Design review of the part built by this model. Coordinates are the model's own, in mm. Round coordinates to 2 decimals unless told otherwise and drop trailing zeros. Write each loop counter-clockwise with the first axis right and the second up, starting at its lowest first coordinate (ties: lowest second). Pieces come first, ordered by that corner, then holes. Notation, with made-up numbers: (20, 16) - (72, 16) arc R27 cw to (72, 53) - close; hole circle Ø9 at (57.25, 77). An arc over 180 degrees is marked (long way). Use one line per item in the form item = value.
```python
from build123d import *

# Parameters (mm, degrees)
SKETCH1_R           = 4.1656
BOSS_EXTRUDE1_DEPTH = 3.175
CUT_EXTRUDE2_DEPTH  = 104.862786526
FILLET1_R           = 12.7


with BuildPart() as part:
    # Sketch1 → Boss-Extrude1 (new body)
    with BuildSketch(Plane.XY):
        with BuildLine():
            Line((-93.98, 26.67), (93.98, 26.67))
            ThreePointArc((93.98, 26.67), (98.470128061, 24.810128061), (100.33, 20.32))
            Line((100.33, 20.32), (100.33, -20.32))
            ThreePointArc((100.33, -20.32), (98.470128061, -24.810128061), (93.98, -26.67))
            Line((93.98, -26.67), (-93.98, -26.67))
            ThreePointArc((-93.98, -26.67), (-98.470128061, -24.810128061), (-100.33, -20.32))
            Line((-100.33, -20.32), (-100.33, 20.32))
            ThreePointArc((-100.33, 20.32), (-98.470128061, 24.810128061), (-93.98, 26.67))
        make_face()
        with Locations((-78.74, 10.922)):
            Circle(SKETCH1_R, mode=Mode.SUBTRACT)
        with Locations((-78.74, -10.922)):
            Circle(SKETCH1_R, mode=Mode.SUBTRACT)
        with Locations(Location((78.74, -10.922, 0), (0, 0, 180))):
            Circle(SKETCH1_R, mode=Mode.SUBTRACT)
        with Locations(Location((78.74, 10.922, 0), (0, 0, 180))):
            Circle(SKETCH1_R, mode=Mode.SUBTRACT)
        with BuildLine():
            Line((-11.43, 13.97), (11.43, 13.97))
            ThreePointArc((11.43, 13.97), (13.226051224, 13.226051224), (13.97, 11.43))
            Line((13.97, 11.43), (13.97, -11.43))
            ThreePointArc((13.97, -11.43), (13.226051224, -13.226051224), (11.43, -13.97))
            Line((11.43, -13.97), (-11.43, -13.97))
            ThreePointArc((-11.43, -13.97), (-13.226051224, -13.226051224), (-13.97, -11.43))
            Line((-13.97, -11.43), (-13.97, 11.43))
            ThreePointArc((-13.97, 11.43), (-13.226051224, 13.226051224), (-11.43, 13.97))
        make_face(mode=Mode.SUBTRACT)
        with BuildLine():
            Line((-52.07, 3.556), (-49.53, 3.556))
            ThreePointArc((-49.53, 3.556), (-45.974, 0), (-49.53, -3.556))
            Line((-49.53, -3.556), (-52.07, -3.556))
            ThreePointArc((-52.07, -3.556), (-55.626, 0), (-52.07, 3.556))
        make_face(mode=Mode.SUBTRACT)
        with BuildLine():
            Line((-26.67, 3.556), (-24.13, 3.556))
            ThreePointArc((-24.13, 3.556), (-20.574, 0), (-24.13, -3.556))
            Line((-24.13, -3.556), (-26.67, -3.556))
            ThreePointArc((-26.67, -3.556), (-30.226, 0), (-26.67, 3.556))
        make_face(mode=Mode.SUBTRACT)
        with BuildLine():
            Line((26.67, 3.556), (24.13, 3.556))
            ThreePointArc((24.13, 3.556), (20.574, 0), (24.13, -3.556))
            Line((24.13, -3.556), (26.67, -3.556))
            ThreePointArc((26.67, -3.556), (30.226, 0), (26.67, 3.556))
        make_face(mode=Mode.SUBTRACT)
        with BuildLine():
            Line((52.07, 3.556), (49.53, 3.556))
            ThreePointArc((49.53, 3.556), (45.974, 0), (49.53, -3.556))
            Line((49.53, -3.556), (52.07, -3.556))
            ThreePointArc((52.07, -3.556), (55.626, 0), (52.07, 3.556))
        make_face(mode=Mode.SUBTRACT)
    extrude(amount=BOSS_EXTRUDE1_DEPTH)

    # Sketch3 → Cut-Extrude2 (cut, through all)
    with BuildSketch(Plane.XY):
        with BuildLine():
            Line((-71.12, 26.67), (-63.409743879, 18.959743879))
            ThreePointArc((-63.409743879, 18.959743879), (-59.289567349, 16.206729937), (-54.429487758, 15.24))
            Line((-54.429487758, 15.24), (-35.650256121, 15.24))
            ThreePointArc((-35.650256121, 15.24), (-30.79017653, 16.206729937), (-26.67, 18.959743879))
            Line((-26.67, 18.959743879), (-18.959743879, 26.67))
            Line((-18.959743879, 26.67), (-71.12, 26.67))
        make_face()
        with BuildLine():
            Line((-71.12, -26.67), (-18.959743879, -26.67))
            Line((-18.959743879, -26.67), (-26.67, -18.959743879))
            ThreePointArc((-26.67, -18.959743879), (-30.79017653, -16.206729937), (-35.650256121, -15.24))
            Line((-35.650256121, -15.24), (-54.429487758, -15.24))
            ThreePointArc((-54.429487758, -15.24), (-59.289567349, -16.206729937), (-63.409743879, -18.959743879))
            Line((-63.409743879, -18.959743879), (-71.12, -26.67))
        make_face()
        with BuildLine():
            Line((71.12, -26.67), (63.409743879, -18.959743879))
            ThreePointArc((63.409743879, -18.959743879), (59.289567349, -16.206729937), (54.429487758, -15.24))
            Line((54.429487758, -15.24), (35.650256121, -15.24))
            ThreePointArc((35.650256121, -15.24), (30.79017653, -16.206729937), (26.67, -18.959743879))
            Line((26.67, -18.959743879), (18.959743879, -26.67))
            Line((18.959743879, -26.67), (71.12, -26.67))
        make_face()
        with BuildLine():
            Line((71.12, 26.67), (18.959743879, 26.67))
            Line((18.959743879, 26.67), (26.67, 18.959743879))
            ThreePointArc((26.67, 18.959743879), (30.79017653, 16.206729937), (35.650256121, 15.24))
            Line((35.650256121, 15.24), (54.429487758, 15.24))
            ThreePointArc((54.429487758, 15.24), (59.289567349, 16.206729937), (63.409743879, 18.959743879))
            Line((63.409743879, 18.959743879), (71.12, 26.67))
        make_face()
    extrude(amount=CUT_EXTRUDE2_DEPTH, mode=Mode.SUBTRACT)

    # Fillet1
    fillet1_edges = [part.edges().sort_by_distance(p)[0] for p in [
        (-18.959743879, 26.67, 1.5875),
        (-71.12, 26.67, 1.5875),
        (-71.12, -26.67, 1.5875),
        (-18.959743879, -26.67, 1.5875),
        (71.12, 26.67, 1.5875),
        (18.959743879, 26.67, 1.5875),
        (18.959743879, -26.67, 1.5875),
        (71.12, -26.67, 1.5875),
    ]]
    fillet(fillet1_edges, radius=FILLET1_R)


solid = part.part
```
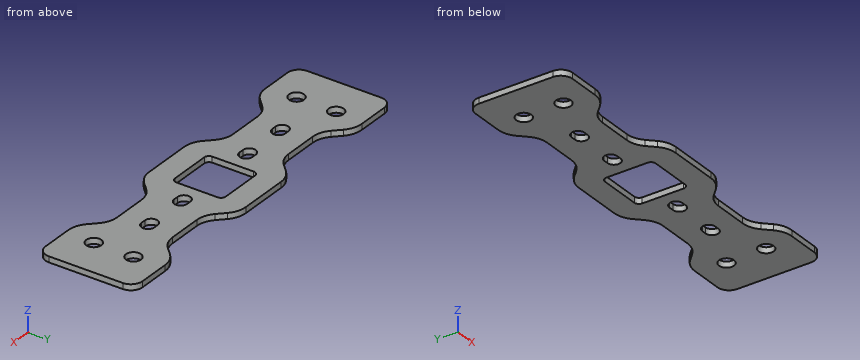
Q1. We need section D-D on x = -32. Write out the cut boundary in (y, z) (3 decimals).
Calculated:
outline = (-15.776, 0) - (15.776, 0) - (15.776, 3.175) - (-15.776, 3.175) - close
Q2. We need section B-B on y = 0. Write out the cut boundary in (x, z) (3 decimals).
Calculated:
outline = (-100.33, 0) - (-55.626, 0) - (-55.626, 3.175) - (-100.33, 3.175) - close; (-45.974, 0) - (-30.226, 0) - (-30.226, 3.175) - (-45.974, 3.175) - close; (-20.574, 0) - (-13.97, 0) - (-13.97, 3.175) - (-20.574, 3.175) - close; (13.97, 0) - (20.574, 0) - (20.574, 3.175) - (13.97, 3.175) - close; (30.226, 0) - (45.974, 0) - (45.974, 3.175) - (30.226, 3.175) - close; (55.626, 0) - (100.33, 0) - (100.33, 3.175) - (55.626, 3.175) - close
Q3. We need section A-A on x = -78.74. Write out the cut boundary in (y, z) (3 decimals).
Calculated:
outline = (-26.67, 0) - (-15.088, 0) - (-15.088, 3.175) - (-26.67, 3.175) - close; (-6.756, 0) - (6.756, 0) - (6.756, 3.175) - (-6.756, 3.175) - close; (15.088, 0) - (26.67, 0) - (26.67, 3.175) - (15.088, 3.175) - close
Q4. We need section C-C on z = 2.45. State how many separate pieces and enclosed holes the cut face has, then the cut area to 3 significant figures.
Calculated:
separate_pieces = 1
enclosed_holes = 9
area = 7,580 mm2
Q5. To check wall thickness, follow line 1 along Y through (x, z) = (78.74, 2); line 2 along X through (y, z) = (13, 3); line 3 along X through (y, z) = (2.5, 0.6). State the ranges of each line that lie inside material, in increasing order. Write a range as from..to.
Calculated:
line_1 = -26.67..-15.09, -6.76..6.76, 15.09..26.67
line_2 = -100.33..-82.35, -75.13..-13.43, 13.43..75.13, 82.35..100.33
line_3 = -100.33..-54.6, -47..-29.2, -21.6..-13.97, 13.97..21.6, 29.2..47, 54.6..100.33
Q6. For P1, Ø1.6, axis at x = -45, z = 1.5, coming from the +Y side; P2, Ø1.3, axis at x = -25.5, z = 1.5, coming from the -Y side, all flat-tipped, find the tip position at first contact; note any pin that passes through.
Calculated:
P1 = 15.24
P2 = -20.78
